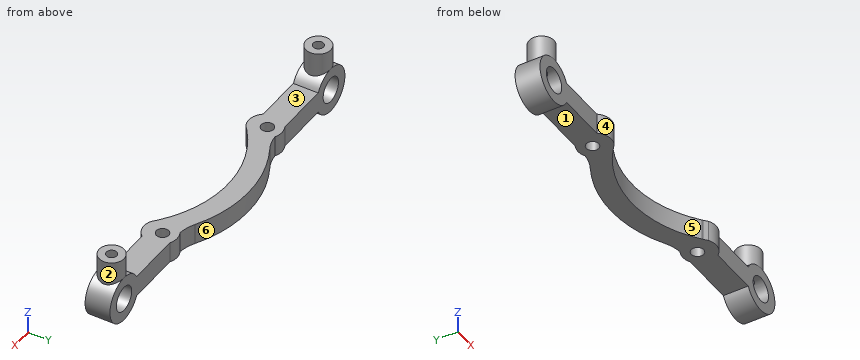
```python
from build123d import *

# Parameters (mm, degrees)
SKETCH1_W                       = 71
SKETCH1_H                       = 6
BOSS_EXTRUDE1_DEPTH             = 5
SKETCH2_R                       = 1.5
CUT_EXTRUDE1_DEPTH              = 36.975686234
SKETCH3_R                       = 4
SKETCH3_R_2                     = 1.5
BOSS_EXTRUDE2_DEPTH             = 5
BOSS_EXTRUDE4_DEPTH             = 5
SKETCH5_R                       = 28
CUT_EXTRUDE3_DEPTH              = 5
FILLET1_R                       = 10
BOSS_EXTRUDE5_REACH             = 38.732
SKETCH6_R                       = 5.5
SKETCH6_R_2                     = 3
BOSS_EXTRUDE5_DIRECTION_2_REACH = 38.732
BOSS_EXTRUDE6_START             = -0.890228
SKETCH7_R                       = 3
SKETCH7_R_2                     = 1.25
BOSS_EXTRUDE6_DEPTH             = 5.890228
CUT_EXTRUDE4_START              = -5
SKETCH8_R                       = 1.25
CUT_EXTRUDE4_DEPTH              = 5
MIRROR7_OUTLINE_W               = 3
MIRROR7_OUTLINE_H               = 5.890504749
CUT_EXTRUDE5_REACH              = 51.262
CUT_EXTRUDE5_END_RADIUS         = 3
SKETCH9_R                       = 1.25


# Read off the part's stored shape, not the designer's step: Mirror7
with BuildPart() as part:
    # Sketch1 → Boss-Extrude1 (new body)
    with BuildSketch(Plane.XY):
        Rectangle(SKETCH1_W, SKETCH1_H)
    extrude(amount=BOSS_EXTRUDE1_DEPTH)

    # Sketch2 → Cut-Extrude1 (cut, through all)
    with BuildSketch(Plane.XY):
        with Locations((20.5, 0)):
            Circle(SKETCH2_R)
        with Locations((-20.5, 0)):
            Circle(SKETCH2_R)
    extrude(amount=CUT_EXTRUDE1_DEPTH, mode=Mode.SUBTRACT)

    # Sketch3 → Boss-Extrude2 (add)
    with BuildSketch(Plane.XY):
        with Locations((20.5, -0.5)):
            Circle(SKETCH3_R)
        with Locations((20.5, 0)):
            Circle(SKETCH3_R_2, mode=Mode.SUBTRACT)
    boss_extrude2 = extrude(amount=BOSS_EXTRUDE2_DEPTH)

    # Mirror1: Boss-Extrude2 across plane
    add(boss_extrude2.mirror(Plane(origin=(0, 0, 0), x_dir=(0, 0, 1), z_dir=(1, 0, 0))))

    # Sketch4 → Boss-Extrude4 (add)
    with BuildSketch(Plane.XY):
        with BuildLine():
            Line((16.583123952, 3), (-16.583123952, 3))
            ThreePointArc((-16.583123952, 3), (0, 8), (16.583123952, 3))
        make_face()
    extrude(amount=BOSS_EXTRUDE4_DEPTH)

    # Sketch5 → Cut-Extrude3 (cut)
    with BuildSketch(Plane.XY):
        with Locations((0, -25)):
            Circle(SKETCH5_R)
    extrude(amount=CUT_EXTRUDE3_DEPTH, mode=Mode.SUBTRACT)

    # Fillet1
    # the kernel refuses this fillet: 10 mm, written as the material it adds along each edge
    with BuildSketch(Plane(origin=(-16.583123952, 3, 0), x_dir=(-1, 0, 0), z_dir=(0, 0, 1))) as fillet1_piece_1:
        with BuildLine():
            CenterArc((2.85012487, -9.962105775), FILLET1_R, 94.989550063, 24.077396017)
            Line((-2.008187335, -1.221579331), (-2.105353579, -1.046768802))
            ThreePointArc((-2.105353579, -1.046768802), (-1.096064984, -0.459595529), (-0.11055416, 0.166666667))
            Line((-0.11055416, 0.166666667), (0, 0.2))
            ThreePointArc((0, 0.2), (0.990192188, 0.2), (1.962989565, 0.199242115))
            Line((1.962989565, 0.199242115), (1.980384375, 0))
        make_face()
    extrude(amount=5)
    with BuildSketch(Plane(origin=(16.583123952, 3, 0), x_dir=(-0.8543488432646742, 0.5196999653764787, 0), z_dir=(0, 0, 1))) as fillet1_piece_2:
        with BuildLine():
            CenterArc((2.74230514, -9.992323342), FILLET1_R, 92.245181841, 24.077396017)
            Line((-1.6919391, -1.029205691), (-1.780623985, -0.849943338))
            ThreePointArc((-1.780623985, -0.849943338), (-0.949909543, -0.343733077), (-0.103939993, 0.170869769))
            Line((-0.103939993, 0.170869769), (0.007835158, 0.199846467))
            ThreePointArc((0.007835158, 0.199846467), (1.175273632, 0.176970025), (2.342712105, 0.199846467))
            Line((2.342712105, 0.199846467), (2.350547263, 0))
        make_face()
    extrude(amount=5)

    # Boss-Extrude5: up to this face of the body (flat: up to its plane)
    boss_extrude5_end = Plane(part.part.faces().sort_by_distance((28.968245837, 3, 2.5))[0])
    # Sketch6 → Boss-Extrude5 (add, up to the picked face)
    with BuildSketch(Plane(origin=(0, 0, 0), x_dir=(1, 0, 0), z_dir=(0, 1, 0)), mode=Mode.PRIVATE) as boss_extrude5_sk1:
        with Locations((40.398979486, -2.5)):
            Circle(SKETCH6_R)
        with Locations(Location((40.398979486, -2.5, 0), (0, 0, 90))):
            Circle(SKETCH6_R_2, mode=Mode.SUBTRACT)
    boss_extrude5_tool1 = split(extrude(boss_extrude5_sk1.sketch, amount=BOSS_EXTRUDE5_REACH, mode=Mode.PRIVATE), bisect_by=boss_extrude5_end, keep=Keep.BOTH, mode=Mode.PRIVATE)
    boss_extrude5 = boss_extrude5_tool1.solids().sort_by(Axis((35.054543, 0, 2.5), (0, 1, 0)))[0]
    add(boss_extrude5)

    # Boss-Extrude5 direction 2: up to this face of the body (flat: up to its plane)
    boss_extrude5_direction_2_end = Plane(part.part.faces().sort_by_distance((29.5612495, -3, 2.5))[0])
    # Sketch6 → Boss-Extrude5 direction 2 (add, up to the picked face)
    with BuildSketch(Plane(origin=(0, 0, 0), x_dir=(1, 0, 0), z_dir=(0, 1, 0)), mode=Mode.PRIVATE) as boss_extrude5_direction_2_sk1:
        with Locations((40.398979486, -2.5)):
            Circle(SKETCH6_R)
        with Locations(Location((40.398979486, -2.5, 0), (0, 0, 90))):
            Circle(SKETCH6_R_2, mode=Mode.SUBTRACT)
    boss_extrude5_direction_2_tool1 = split(extrude(boss_extrude5_direction_2_sk1.sketch, amount=-BOSS_EXTRUDE5_DIRECTION_2_REACH, mode=Mode.PRIVATE), bisect_by=boss_extrude5_direction_2_end, keep=Keep.BOTH, mode=Mode.PRIVATE)
    boss_extrude5_direction_2 = boss_extrude5_direction_2_tool1.solids().sort_by(Axis((35.054543, 0, 2.5), (0, -1, 0)))[0]
    add(boss_extrude5_direction_2)

    # Sketch7 → Boss-Extrude6 (add)
    with BuildSketch(Plane.XY.offset(8).offset(BOSS_EXTRUDE6_START)):
        with Locations(Location((40.398979486, 0, 0), (0, 0, 269.999999959))):
            Circle(SKETCH7_R)
        with Locations((40.398979486, 0)):
            Circle(SKETCH7_R_2, mode=Mode.SUBTRACT)
    extrude(amount=BOSS_EXTRUDE6_DEPTH)

    # Sketch8 → Cut-Extrude4 (cut)
    with BuildSketch(Plane.XY.offset(8).offset(CUT_EXTRUDE4_START)):
        with Locations((40.398979486, 0)):
            Circle(SKETCH8_R)
    extrude(amount=CUT_EXTRUDE4_DEPTH, mode=Mode.SUBTRACT)

    # Mirror5: Boss-Extrude5, Boss-Extrude5 direction 2 across plane
    add(boss_extrude5.mirror(Plane(origin=(0, 0, 0), x_dir=(0, 0, 1), z_dir=(1, 0, 0))))
    add(boss_extrude5_direction_2.mirror(Plane(origin=(0, 0, 0), x_dir=(0, 0, 1), z_dir=(1, 0, 0))))

    # Mirror7 outline → Mirror7 (revolve)
    with BuildSketch(Plane(origin=(-40.398979486, 0, 0), x_dir=(1, 0, 0), z_dir=(0, -1, 0))):
        with Locations((1.5, 10.054747625)):
            Rectangle(MIRROR7_OUTLINE_W, MIRROR7_OUTLINE_H)
    revolve(axis=Axis((-40.398979486, 0, 0), (0, 0, 1)))

    # Cut-Extrude5: up to this cylinder (the profile starts outside it)
    cut_extrude5_end = Plane(origin=(-40.398979486, 0, 2.5), z_dir=(0, -1, 0)) * Cylinder(CUT_EXTRUDE5_END_RADIUS, 109.524, mode=Mode.PRIVATE)
    # Sketch9 → Cut-Extrude5 (cut, up to the surface)
    with BuildSketch(Plane.XY.offset(13), mode=Mode.PRIVATE) as cut_extrude5_sk1:
        with Locations((-40.398979486, 0)):
            Circle(SKETCH9_R)
    cut_extrude5_tool1 = extrude(cut_extrude5_sk1.sketch, amount=-CUT_EXTRUDE5_REACH, mode=Mode.PRIVATE) - cut_extrude5_end
    add(cut_extrude5_tool1.solids().sort_by_distance((-40.398979, 0, 13))[0], mode=Mode.SUBTRACT)


solid = part.part
```
Geometry check sheet. Reference: the model listing, model coordinates, mm. Face numbers are marked on the shaded views. A direction names the side the tool comes from. Round coordinates to 2 decimals unless told otherwise and drop trailing zeros. Loops run counter-clockwise (first coordinate to the right, second up) from the corner with the lowest first, then second, coordinate; pieces in that order, holes last. Notation, with made-up numbers: (44, 5.5) - (70, 5.5) arc R11 ccw to (70, 10.5) - close; hole circle Ø2 at (30.5, 57.25). An arc over 180 degrees is marked (long way). Use a Markdown table: item, result.
Q1. Access from +Z, -Z, +X, -X, +Y, -Y to the whole of each face (thin tool, end or side, straight path). Record for the marked faces 1, 2 and 3.
Solutions:
| item | result |
|---|---|
| face 1 | -Z, +Y, -Y |
| face 2 | +Z |
| face 3 | +Z, +Y, -Y |
Q2. Cross-section at D-D on x = 29. Record the cut outline in (y, z).
Solutions:
| item | result |
|---|---|
| outline | (-3, 0) - (3, 0) - (3, 5) - (-3, 5) - close |
Q3. Go/stop test with flat-tipped pins: P1, Ø3, axis at x = -21.5, y = 4.5, coming from the +Z side; P2, Ø8, axis at x = -40.4, z = 2.5, coming from the +Y side; P3, Ø9, axis at x = 39, z = 2, coming from the -Y side. Record where each tip stops, or that it passes through.
Solutions:
| item | result |
|---|---|
| P1 | stops at z = 5 |
| P2 | stops at y = 3 |
| P3 | stops at y = -3 |
Q4. Cross-section at C-C on y = 6.5. Record the cut outline in (x, z), plus the area to 3 significant figures.
Solutions:
| item | result |
|---|---|
| outline | (-9.37, 0) - (9.37, 0) - (9.37, 5) - (-9.37, 5) - close |
| area | 93.7 mm2 |
Q5. Draft check along X on the marked faces 4, 5 and 6. Enter one of: released by +X, released by -X, zero draft, split by the parting line, or undercut.
Solutions:
| item | result |
|---|---|
| face 4 | undercut |
| face 5 | undercut |
| face 6 | split by the parting line |
Q6. Material ranges on line 1 (X direction, y = -0.25, z = 5.5); line 2 (X direction, y = -1, z = 2.5); line 3 (Z direction, x = -17, y = 0.5), recorded low to high.
Solutions:
| item | result |
|---|---|
| line 1 | x = -45.01 to -41.62, -39.17 to -35.79, 35.79 to 39.17, 41.62 to 45.01 |
| line 2 | x = -45.9 to -43.4, -37.4 to -21.62, -19.38 to -14.42, 14.42 to 19.38, 21.62 to 37.4, 43.4 to 45.9 |
| line 3 | z = 0 to 5 |
Q7. Cross-section at B-B on z = 2.5. State how many separate pieces and enclosed holes the cut face has, plus the area to 3 significant figures.
Solutions:
| item | result |
|---|---|
| separate pieces | 3 |
| enclosed holes | 2 |
| area | 452 mm2 |
Q8. Cross-section at A-A on x = -20.5. Record the cut outline in (y, z), plus the area to 3 significant figures.
Solutions:
| item | result |
|---|---|
| outline | (-4.5, 0) - (-1.5, 0) - (-1.5, 5) - (-4.5, 5) - close; (1.5, 0) - (3.5, 0) - (3.5, 5) - (1.5, 5) - close |
| area | 25.0 mm2 |
